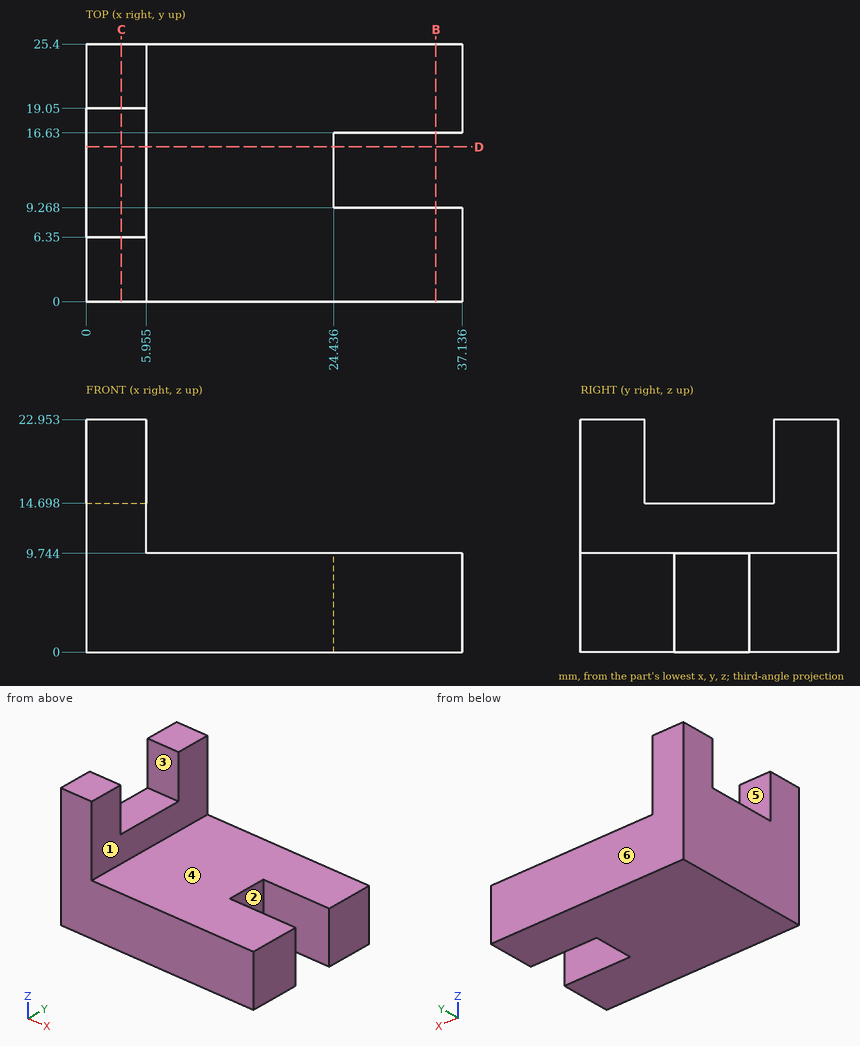
Check sheet for the drawn part. Datum: minimum x, y, z corner. Units: mm. A direction names the side the tool comes from. Round coordinates to 2 decimals unless told otherwise and drop trailing zeros. Loops run counter-clockwise (first coordinate to the right, second up) from the corner with the lowest first, then second, coordinate; pieces in that order, holes last.
Item 1: Cross-section at C-C on x = 3.5. Record the boundary of the cut face in (y, z), then the cut area to 3 significant figures.
Item 2: Thickness scan on line 1 (Y direction, x = 33, z = 3); line 2 (Z direction, x = 15, y = 13.75); line 3 (X direction, y = 22.25, z = 20.25) (1 decimal). Record the ranges inside material, lowest first.
Item 3: Mould release check, pull along Y, two halves, no side actions. Record for the marked faces 4, 5 and 6: pulls with the +Y half, pulls with the -Y half, needs draft (parallel to the pull), parting line crosses it, or undercut.
Item 4: Access from +Z, -Z, +X, -X, +Y, -Y to the whole of each face (thin tool, end or side, straight path). Record for the marked faces 1, 2 and 3.
Item 5: Gauge pin test, flat ends, axial feed: pin 1 (1.8 mm diameter, centred on x = 2.5, y = 13, fed in from +Z); pin 2 (8 mm diameter, centred on x = 31.5, y = 10.5, fed in from +Z); pin 3 (6.5 mm diameter, centred on y = 12, z = 17.5, fed in from +X) (1 decimal). Record the tip position at first contact, or that the pin passes through.
Item 6: Cross-section at B-B on x = 34.5. Record the boundary of the cut face in (y, z).
Item 7: Cross-section at D-D on y = 15.25. Record the boundary of the cut face in (x, z) (1 decimal).
Answer sheet:
1. outline: (0, 0) - (25.4, 0) - (25.4, 22.95) - (19.05, 22.95) - (19.05, 14.7) - (6.35, 14.7) - (6.35, 22.95) - (0, 22.95) - close
1. area: 478 mm2
2. line 1: y = 0 to 9.27, 16.63 to 25.4
2. line 2: z = 0 to 9.74
2. line 3: x = 0 to 6
3. face 4: needs draft
3. face 5: undercut
3. face 6: pulls with the +Y half
4. face 1: +Z, +X, +Y, -Y
4. face 2: +Z, -Z, +X
4. face 3: +Z, +X, -X
5. pin 1: stops at z = 14.7
5. pin 2: stops at z = 9.74
5. pin 3: stops at x = 6
6. outline: (0, 0) - (9.27, 0) - (9.27, 9.74) - (0, 9.74) - close; (16.63, 0) - (25.4, 0) - (25.4, 9.74) - (16.63, 9.74) - close
7. outline: (0, 0) - (24.4, 0) - (24.4, 9.7) - (6, 9.7) - (6, 14.7) - (0, 14.7) - close
